Build history of the part. All positions in model axes, mm. Give positions to 0.01 mm unless a question says otherwise; leave off trailing zeros. Loops run counter-clockwise (first coordinate to the right, second up) from the corner with the lowest first, then second, coordinate; pieces in that order, holes last. Notation, with made-up numbers: M 51,25 L 58,25 A27 cw 58,47 Z; hole C 30.25,-40 d6. An arc over 180 degrees is marked long. Answer in a Markdown table with one row per item. Add a question column.
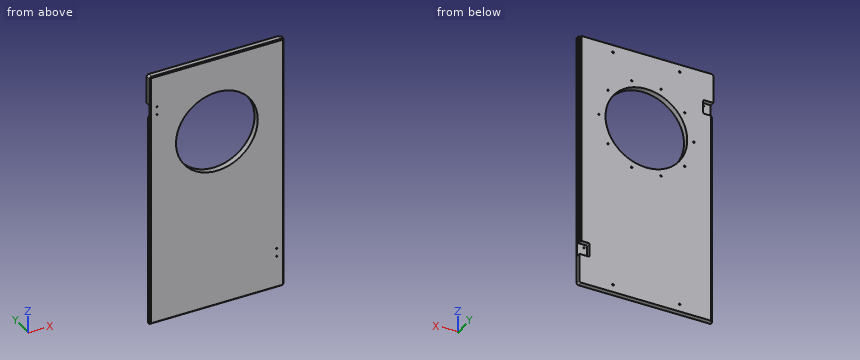
Autodesk Inventor part; units mm, degrees
ref_plane "Work Plane1" through (0, 0, 150) normal (0, 0, 1) x (1, 0, 0)
ref_plane "Work Plane2" through (0, 15.875, 140) normal (0, 1, 0) x (1, 0, 0)
ref_plane "YZ Plane" through (0, 0, 0) normal (1, 0, 0) x (0, 1, 0)
sketch "Sketch1" plane through (0, 0, 0) normal (0, 1, 0) x (-1, 0, 0)
  line L0 (180, 345) -> (-180, 345)
  line L1 (-180, 345) -> (-180, -345)
  line L2 (-180, -345) -> (180, -345)
  line L3 (180, -345) -> (180, 345)
  line L4 (180, 345) -> (-180, -345) construction
  line L5 (-180, 345) -> (180, -345) construction
  point P0 (0, 0)
  dimension "d0" = 360
  dimension "d1" = 690
extrude "Extrusion1" add sketch "Sketch1" along normal blind 15.875
sketch "Sketch2" plane through (0, 15.875, 0) normal (0, 1, 0) x (1, 0, 0)
  circle A0 centre (0, -140) radius 110
  line L0 (-180, -345) -> (180, -345)
  circle A1 centre (0, -140) radius 135
  point P0 (0, 0)
  dimension "d4" = 205
  dimension "d5" = 220
  dimension "d8" = 270
extrude "Extrusion2" cut sketch "Sketch2" against normal through all contours A0
ref_plane "Work Plane1" through (0, 0, 150) normal (0, 0, 1) x (1, 0, 0)
sketch "Sketch6" plane through (0, 15.875, 0) normal (0, 1, 0) x (1, 0, 0)
  line L0 (89.6938, -325) -> (-89.6938, -325)
  line L1 (-89.6938, -325) -> (-89.6938, 325)
  line L2 (-89.6938, 325) -> (89.6938, 325)
  line L3 (89.6938, 325) -> (89.6938, -325)
  line L4 (89.6938, -325) -> (-89.6938, 325) construction
  line L5 (-89.6938, -325) -> (89.6938, 325) construction
  point P0 (0, 0)
  dimension "d55" = 179.3875
  dimension "d56" = 650
hole "Hole3" at (89.6938, 15.875, 325) at (-89.6938, 15.875, 325) at (-89.6938, 15.875, -325) at (89.6938, 15.875, -325) direction (0, -1, 0) diameter 4.917 depth 5 tip angle 118
sketch "Sketch7" plane through (0, 15.875, 0) normal (0, 1, 0) x (1, 0, 0)
  circle A0 centre (0, -140) radius 110
  circle A1 centre (0, -140) radius 131.5
  circle A2 centre (0, -140) radius 135
  point P0 (0, 0)
  dimension "d64" = 263
  dimension "d65" = 270
ref_plane "Work Plane2" through (0, 15.875, 140) normal (0, 1, 0) x (1, 0, 0)
sketch "Sketch8" plane through (0, 15.875, 140) normal (0, 1, 0) x (1, 0, 0)
  circle A0 centre (0, 0) radius 131.5
  circle A1 centre (0, 0) radius 127.5
  circle A2 centre (127.5, 0) radius 2
  circle A3 centre (103.1497, 74.9426) radius 2
  circle A4 centre (39.3997, 121.2597) radius 2
  circle A5 centre (-39.3997, 121.2597) radius 2
  circle A6 centre (-103.1497, 74.9426) radius 2
  circle A7 centre (-127.5, 0) radius 2
  circle A8 centre (-103.1497, -74.9426) radius 2
  circle A9 centre (-39.3997, -121.2597) radius 2
  circle A10 centre (39.3997, -121.2597) radius 2
  circle A11 centre (103.1497, -74.9426) radius 2
  point P0 (0, 140)
  dimension "d68" = 255
  dimension "d69" = 4
  dimension "d72" = 360
hole "Hole4" at (127.5, 15.875, 140) at (103.1497, 15.875, 214.9426) at (39.3997, 15.875, 261.2597) at (-39.3997, 15.875, 261.2597) at (-103.1497, 15.875, 214.9426) at (-127.5, 15.875, 140) at (-103.1497, 15.875, 65.0574) at (-39.3997, 15.875, 18.7403) at (39.3997, 15.875, 18.7403) at (103.1497, 15.875, 65.0574) direction (0, -1, 0) diameter 4.134 depth 10 tip angle 118
sketch "Sketch9" plane through (0, 15.875, 0) normal (0, 1, 0) x (1, 0, 0)
  line L0 (180, -345) -> (180, 345)
  line L1 (180, 266) -> (156, 266)
  line L2 (153, 263) -> (153, 231)
  line L3 (156, 228) -> (180, 228)
  line L4 (180, 228) -> (180, 266)
  line L5 (-180, 345) -> (-180, -345)
  line L6 (-180, -266) -> (-156, -266)
  line L7 (-153, -263) -> (-153, -231)
  line L8 (-156, -228) -> (-180, -228)
  line L9 (-180, -228) -> (-180, -266)
  line L10 (180, 345) -> (-180, 345)
  line L11 (-180, -345) -> (180, -345)
  arc A0 (153, 231) -> (156, 228) centre (156, 231) ccw
  arc A1 (156, 266) -> (153, 263) centre (156, 263) ccw
  arc A2 (-156, -266) -> (-153, -263) centre (-156, -263) ccw
  arc A3 (-153, -231) -> (-156, -228) centre (-156, -231) ccw
  point P0 (0, 0)
  point P1 (153, 228)
  point P2 (153, 266)
  point P3 (-153, -228)
  point P4 (-153, -266)
  dimension "d82" = 27
  dimension "d83" = 27
  dimension "d84" = 38
  dimension "d85" = 38
  dimension "d86" = 79
  dimension "d87" = 79
  dimension "d95" = 3
  dimension "d96" = 3
fillet "Fillet2" radius 5 2 edges at (180, 7.9375, -345) (-180, 7.9375, 345)
extrude "Extrusion7" cut sketch "Sketch9" against normal blind 12.575 contours L3 A0 L2 A1 L1 L0 | L5 L8 A3 L7 A2 L6
sketch "Sketch10" plane through (0, 15.875, 0) normal (0, 1, 0) x (1, 0, 0)
  line L0 (-180, -266) -> (-180, -228)
  line L1 (175, 345) -> (-180, 345)
  line L2 (-180, -228) -> (-174, -228)
  line L3 (-174, -228) -> (-174, 345)
  line L4 (-174, 345) -> (-180, 345)
  line L5 (-180, 345) -> (-180, -228)
  line L6 (180, 228) -> (156, 228)
  line L7 (-175, -345) -> (180, -345)
  line L8 (180, 228) -> (174, 228)
  line L9 (174, 228) -> (174, -345)
  line L10 (174, -345) -> (180, -345)
  line L11 (180, -345) -> (180, 228)
  point P0 (0, 0)
  point P1 (180, -345)
  dimension "d99" = 6
  dimension "d100" = 6
extrude "Extrusion8" cut sketch "Sketch10" against normal blind 3.1
chamfer "Chamfer3" distance 2 distance2 3.5 1 edges at (180, 12.775, 58.5) measured on face at (180, 5.3583, 154)
chamfer "Chamfer4" distance 3.5 distance2 2 1 edges at (-180, 12.775, -58.5) measured on face at (-180, 5.3583, -154)
sketch "Sketch11" plane through (0, 3.3, 0) normal (0, 1, 0) x (1, 0, 0)
  circle A0 centre (-161, -236) radius 1.65
  circle A1 centre (-161, -258) radius 1.65
  circle A2 centre (161, 258) radius 1.65
  circle A3 centre (161, 236) radius 1.65
  line L0 (-180, -266) -> (-180, -228)
  line L1 (-156, -266) -> (-180, -266)
  line L2 (174, 228) -> (156, 228)
  line L3 (180, 266) -> (180, 228)
  point P0 (0, 0)
  dimension "d109" = 19
  dimension "d110" = 8
  dimension "d111" = 22
  dimension "d112" = 19
  dimension "d113" = 3.3
  dimension "d114" = 3.3
  dimension "d115" = 3.3
  dimension "d116" = 3.3
  dimension "d118" = 8
  dimension "d119" = 22
  dimension "d120" = 19
  dimension "d121" = 19
hole "Hole5" at (-161, 3.3, 258) at (-161, 3.3, 236) at (161, 3.3, -236) at (161, 3.3, -258) direction (0, -1, 0) diameter 3.242 end through all
chamfer "Chamfer5" distance 0.35 angle 45 4 edges at (-161, 3.3, 256.379) (-161, 3.3, 234.379) (161, 3.3, -259.621) (161, 3.3, -237.621)
chamfer "Chamfer6" distance 2.5 angle 45 3 edges at (178.5355, 0, -343.5355) (-2.5, 0, -345) (180, 0, 2.5)
chamfer "Chamfer7" distance 2.5 angle 45 3 edges at (-178.5355, 0, 343.5355) (1.25, 0, 345) (-180, 0, -1.25)
properties part number "Updated Cover"
(1) Wall check: line 1 (Z direction, x = 127.5, y = 8.5); line 2 (Z direction, x = 79, y = 9.25); line 3 (Z direction, x = -160, y = 1.25). Give the ranges that are in metal, low to high.
(2) Slice it at C-C, the plane x = 9.5. Give the cut face in (y, z) (3 decimals).
(3) Pin check, flat tips, straight feed: pin 1 (6.5 mm diameter, centred on x = 39.4, z = 18.74, fed in from -Y); pin 2 (4.5 mm diameter, centred on x = -176.5, z = -65, fed in from +Y) (3 decimals); pin 3 (2.5 mm diameter, centred on x = -103.15, z = 65.06, fed in from +Y); pin 4 (13.5 mm diameter, centred on x = 168.5, z = -247.5, fed in from +Y). Stop position of each tip, or through.
(4) Slice it at B-B, the plane x = 52. Give the cut face in (y, z) (3 decimals).
(5) Slice it at A-A, the plane z = 182.5. Give the cut face in (x, y) (3 decimals), then the cut area to 3 significant figures.
Solution:
| question | item | result |
|---|---|---|
| 1 | line 1 | -345 to 137.93, 142.07 to 345 |
| 1 | line 2 | -345 to 63.46, 216.54 to 345 |
| 1 | line 3 | -343.75 to 234.72, 237.28 to 256.72, 259.28 to 343.75 |
| 2 | outline | M 0,-342.5 L 2.5,-345 L 15.875,-345 L 15.875,30.411 L 0,30.411 Z; M 0,249.589 L 15.875,249.589 L 15.875,345 L 2.5,345 L 0,342.5 Z |
| 3 | pin 1 | y = 0 |
| 3 | pin 2 | y = 12.775 |
| 3 | pin 3 | y = 5.39 |
| 3 | pin 4 | y = 3.3 |
| 4 | outline | M 0,-342.5 L 2.5,-345 L 15.875,-345 L 15.875,43.067 L 0,43.067 Z; M 0,236.933 L 15.875,236.933 L 15.875,345 L 2.5,345 L 0,342.5 Z |
| 5 | outline | M -180,2.5 L -177.5,0 L -101.458,0 L -101.458,15.875 L -174,15.875 L -174,12.775 L -178,12.775 L -180,9.275 Z; M 101.458,0 L 177.5,0 L 180,2.5 L 180,10.775 L 176.5,12.775 L 174,12.775 L 174,15.875 L 101.458,15.875 Z |
| 5 | area | 2,440 mm^2 |
